from build123d import *
from build123d.topology import SkipClean

# Parameters (mm, degrees)
BOSS_EXTRUDE1_DEPTH      = 4
SKETCH4_R                = 8
BOSS_EXTRUDE2_DEPTH      = 2
BOSS_EXTRUDE3_DEPTH      = 3
F_3_0_3_DIAMETER_HOLE1_D = 3
F_6_0_6_DIAMETER_HOLE1_D = 6


with BuildPart() as part:
    # Sketch1 → Boss-Extrude1 (new body)
    with BuildSketch(Plane.XY):
        with BuildLine():
            Line((3.123869731, 7.364878676), (12, 3.6))
            Line((12, 3.6), (23.9, 3.6))
            ThreePointArc((23.9, 3.6), (27.5, 0), (23.9, -3.6))
            Line((23.9, -3.6), (12, -3.6))
            Line((12, -3.6), (3.123869731, -7.364878676))
            ThreePointArc((3.123869731, -7.364878676), (-8, 0), (3.123869731, 7.364878676))
        make_face()
    extrude(amount=BOSS_EXTRUDE1_DEPTH)

    # Sketch4 → Boss-Extrude2 (add)
    with SkipClean():  # the faces are left unmerged after this step: merging them gives an invalid solid
        with BuildSketch(Plane.XY.offset(4)):
            with Locations(Location((0, 0, 0), (0, 0, 67.015399011))):
                Circle(SKETCH4_R)
        extrude(amount=BOSS_EXTRUDE2_DEPTH)

    # Sketch5 → Boss-Extrude3 (add)
    with SkipClean():  # the faces are left unmerged after this step: merging them gives an invalid solid
        with BuildSketch(Plane.XY.offset(4)):
            with BuildLine():
                Line((23.9, -2.5), (19.9, -2.5))
                ThreePointArc((19.9, -2.5), (17.4, 0), (19.9, 2.5))
                Line((19.9, 2.5), (23.9, 2.5))
                ThreePointArc((23.9, 2.5), (26.4, 0), (23.9, -2.5))
            make_face()
        extrude(amount=BOSS_EXTRUDE3_DEPTH)

    # Ø3.0 (3) Diameter Hole1 (through all)
    with Locations(Plane(origin=(0, 0, 0), x_dir=(-1, 0, 0), z_dir=(0, 0, -1))):
        with Locations((-23.9, 0), (-19.9, 0)):
            Hole(F_3_0_3_DIAMETER_HOLE1_D / 2)

    # Ø6.0 (6) Diameter Hole1 (through all)
    with Locations(Plane(origin=(0, 0, 0), x_dir=(-1, 0, 0), z_dir=(0, 0, -1))):
        with Locations((0, 0)):
            Hole(F_6_0_6_DIAMETER_HOLE1_D / 2)


solid = part.part
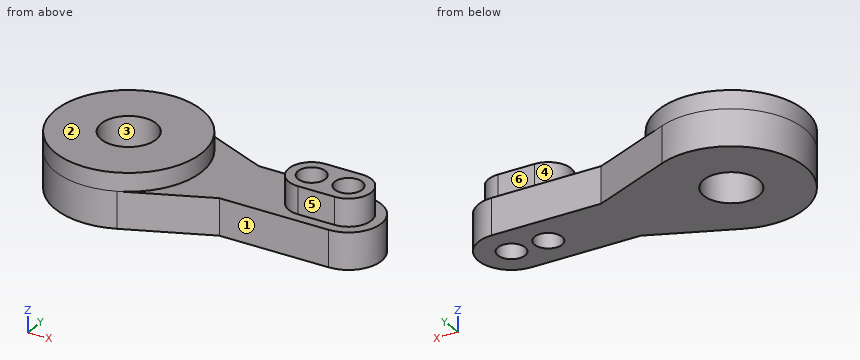
Can you work these out from the model? Positions are in its coordinate system, mm. Face numbers are marked on the shaded views. A direction names the side the tool comes from. Round coordinates to 2 decimals unless told otherwise and drop trailing zeros. Loops run counter-clockwise (first coordinate to the right, second up) from the corner with the lowest first, then second, coordinate; pieces in that order, holes last. Notation, with made-up numbers: (-25, 38) - (23, 38) arc R27 ccw to (23, 74) - close; hole circle Ø5 at (-18, 70). An arc over 180 degrees is marked (long way). Write item = value, one per line. Start each with the question number.
(1) If we mould it in two halves opening along Y, with no side actions, what happens to the marked faces 1, 2 and 3? For each: released by +Y, released by -Y, zero draft, split by the parting line, or undercut.
(2) For P1, Ø4, axis at x = 12, z = 5.5, coming from the +Y side; P2, Ø3, axis at x = 16, z = 3, coming from the +Y side; P3, Ø3.5, axis at x = 22, z = 6, coming from the -Y side, each with a flat end and sliding along its axis, tell me the tip position at first contact or that it passes through.
(3) If we section it at D-D (y = 5.5): Please give me the cut outline in (x, z).
(4) For the marked faces 4, 5 and 6, which set-ups out of +Z, -Z, +X, -X, +Y, -Y let a thin tool reach every point of the face, with its end or its side?
(5) If we section it at A-A (x = 0): Please give me the cut outline in (y, z).
(6) If we section it at C-C (z = 2.25): Please give me the cut outline in (x, y).
(7) If I drill on probe 1 along Y at (x, z) = (23.9, 3); probe 2 along X at (y, z) = (-1, 2.5); probe 3 along X at (y, z) = (-1, 6.5), over which ranges is the centre line in solid material (lowest first)? Write a range as [from, to].
(8) If we section it at B-B (y = 0): Please give me the cut outline in (x, z), and give its area (3 significant figures).
Ans:
q1.face_1 = released by -Y
q1.face_2 = zero draft
q1.face_3 = undercut
q2.P1 = 4.16
q2.P2 = 3.6
q2.P3 = -2.5
q3.outline = (-5.81, 0) - (7.52, 0) - (7.52, 4) - (5.81, 4) - (5.81, 6) - (-5.81, 6) - close
q4.face_4 = +Z
q4.face_5 = +Z, +X, -Y
q4.face_6 = +Z, +X, +Y
q5.outline = (-8, 0) - (-3, 0) - (-3, 6) - (-8, 6) - close; (3, 0) - (8, 0) - (8, 6) - (3, 6) - close
q6.outline = (3.12, -7.36) - (12, -3.6) - (23.9, -3.6) arc R3.6 ccw to (23.9, 3.6) - (12, 3.6) - (3.12, 7.36) arc R8 ccw (long way) to start; hole circle Ø6 at (0, 0); hole circle Ø3 at (19.9, 0); hole circle Ø3 at (23.9, 0)
q7.probe_1 = [-3.6, -1.5], [1.5, 3.6]
q7.probe_2 = [-7.94, -2.83], [2.83, 18.78], [21.02, 22.78], [25.02, 27.36]
q7.probe_3 = [17.61, 18.78], [21.02, 22.78], [25.02, 26.19]
q8.outline = (-8, 0) - (-3, 0) - (-3, 6) - (-8, 6) - close; (3, 0) - (18.4, 0) - (18.4, 7) - (17.4, 7) - (17.4, 4) - (8, 4) - (8, 6) - (3, 6) - close; (21.4, 0) - (22.4, 0) - (22.4, 7) - (21.4, 7) - close; (25.4, 0) - (27.5, 0) - (27.5, 4) - (26.4, 4) - (26.4, 7) - (25.4, 7) - close
q8.area = 123 mm²
